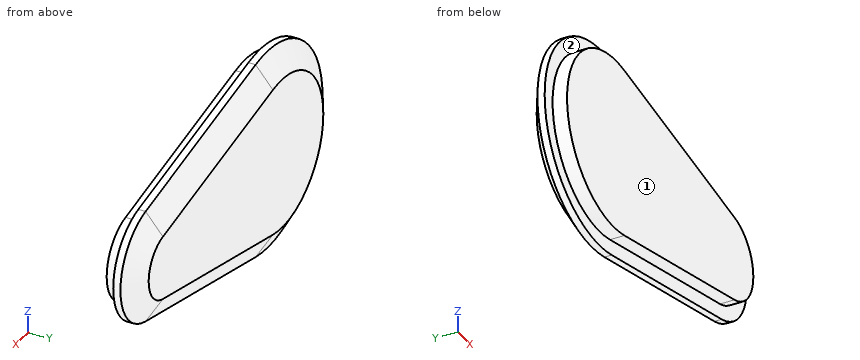
from build123d import *

# Parameters (mm, degrees)
BOSS_EXTRUDE1_DEPTH = 2
BOSS_EXTRUDE2_DEPTH = 1
BOSS_EXTRUDE3_DEPTH = 2
BOSS_EXTRUDE3_TAPER = 60


with BuildPart() as part:
    # Sketch1 → Boss-Extrude1 (new body)
    with BuildSketch(Plane(origin=(0, 0, 0), x_dir=(1, 0, 0), z_dir=(0, 1, 0))):
        with BuildLine():
            Line((2.482758621, 11.740353897), (30.24137931, 5.870176949))
            ThreePointArc((30.24137931, 5.870176949), (35, 0), (30.24137931, -5.870176949))
            Line((30.24137931, -5.870176949), (2.482758621, -11.740353897))
            ThreePointArc((2.482758621, -11.740353897), (-12, 0), (2.482758621, 11.740353897))
        make_face()
    extrude(amount=BOSS_EXTRUDE1_DEPTH)

    # Sketch2 → Boss-Extrude2 (add)
    with BuildSketch(Plane(origin=(0, 2, 0), x_dir=(1, 0, 0), z_dir=(0, 1, 0))):
        with BuildLine():
            Line((30.655172414, 7.826902598), (2.896551724, 13.697079547))
            ThreePointArc((2.896551724, 13.697079547), (-14, 0), (2.896551724, -13.697079547))
            Line((2.896551724, -13.697079547), (30.655172414, -7.826902598))
            ThreePointArc((30.655172414, -7.826902598), (37, 0), (30.655172414, 7.826902598))
        make_face()
    extrude(amount=BOSS_EXTRUDE2_DEPTH)

    # Sketch3 → Boss-Extrude3 (add)
    with BuildSketch(Plane(origin=(0, 3, 0), x_dir=(1, 0, 0), z_dir=(0, 1, 0))):
        with BuildLine():
            Line((30.655172414, 7.826902598), (2.896551724, 13.697079547))
            ThreePointArc((2.896551724, 13.697079547), (-14, 0), (2.896551724, -13.697079547))
            Line((2.896551724, -13.697079547), (30.655172414, -7.826902598))
            ThreePointArc((30.655172414, -7.826902598), (37, 0), (30.655172414, 7.826902598))
        make_face()
    extrude(amount=BOSS_EXTRUDE3_DEPTH, taper=BOSS_EXTRUDE3_TAPER)


solid = part.part
Geometry: final body of the model. Coordinates: model frame, mm. Face numbers are marked on the shaded views. A direction names the side the tool comes from. Coordinates: 2 decimals unless noted, no trailing zeros. Order: outer loops, then holes, each group sorted by start corner. A loop starts at its lowest first (then second) coordinate and runs counter-clockwise, first axis right, second up. Notation, with made-up numbers: M 57,-6.5 L 63,-6.5 A5 cw 63,-0.5 Z; hole C 32,-37.5 d7. An arc over 180 degrees is marked long. One line per question, with ' | ' between items. Start each with the question number.
Item 1: Cut plane C-C, the plane y = 0.75. Return the cut outline in (x, z).
Item 2: Cut plane B-B, the plane x = 0. Return the cut outline in (y, z).
Item 3: Pin query (flat end, axial travel): pin 1 Ø4 at (x, z) = (18.5, 11) entering from -Y; pin 2 Ø3 at (y, z) = (3, -5.5) entering from +X. Return the tip coordinate at first contact, or that it passes through.
Item 4: Ray query, probe 1 along Z at (x, y) = (1.5, 4.1); probe 2 along Y at (x, z) = (24.5, 9); probe 3 along Z at (x, y) = (30, 0.6). Return the intervals inside material, ascending. Write a range as [from, to].
Item 5: Set-up query: the marked faces 1 and 2. Return all of +Z, -Z, +X, -X, +Y, -Y with unobstructed straight access to the full face (end or side cutting, diameter ignored); none if empty.
Item 6: Cut plane A-A, the plane z = 0. Return the cut outline in (x, y).
A:
1) outline: M 2.48,-11.74 L 30.24,-5.87 A6 ccw 30.24,5.87 L 2.48,11.74 A12 ccw long Z
2) outline: M 0,-12 L 2,-12 L 2,-14 L 3,-14 L 5,-10.54 L 5,10.54 L 3,14 L 2,14 L 2,12 L 0,12 Z
3) pin 1: stops at y = 2 | pin 2: stops at x = 35.93
4) probe 1: z = [-12, 12] | probe 2: y = [2, 3.07] | probe 3: z = [-5.92, 5.92]
5) face 1: +Z, -Z, +X, -X, -Y | face 2: -Y
6) outline: M -14,2 L -12,2 L -12,0 L 35,0 L 35,2 L 37,2 L 37,3 L 33.54,5 L -10.54,5 L -14,3 Z
